Design review of the part built by this model. Coordinates are the model's own, in mm. Face numbers are marked on the shaded views. A direction names the side the tool comes from. Round coordinates to 2 decimals unless told otherwise and drop trailing zeros. Write each loop counter-clockwise with the first axis right and the second up, starting at its lowest first coordinate (ties: lowest second). Pieces come first, ordered by that corner, then holes. Notation, with made-up numbers: (12, 27.25) -> (43, 27.25) arc R4 cw to (43, 32.25) -> close; hole circle Ø11 at (8, 45.5). An arc over 180 degrees is marked (long way). Write item = value, one per line. Start each with the question number.
Item 1: Add section B-B, the plane y = -20. State the section outline as (x, z) points, then the cut area to 3 significant figures.
Item 2: Add section D-D, the plane y = 10. State the section outline as (x, z) points, then the cut area to 3 significant figures.
Item 3: Add section C-C, the plane x = 23. State the section outline as (y, z) points.
Item 4: Add section A-A, the plane x = 0. State the section outline as (y, z) points.
Item 5: For pin 1 Ø6 at (x, z) = (38, 29.5) entering from -Y, flat-tipped, find the tip position at first contact; note if it passes through.
Item 6: To check wall thickness, follow L1, parallel to Z at x = 25, y = -10.5; L2, parallel to Y at x = -21.5, z = 19.5; L3, parallel to Y at x = -13, z = 6.5. State the ranges of each line that lie inside material, in increasing order.
Item 7: Mouldability with a two-part tool opening along Y and no side actions: class the marked faces 1, 2, 3 and 4 as released by +Y, released by -Y, zero draft, split by the parting line, or undercut.
Item 8: Machinability: for the marked faces 5 and 6, which of the approach directions +Z, -Z, +X, -X, +Y, -Y give a long, thin tool a straight path to every point of the face, cutting with its end or side? Answer none if there is none.
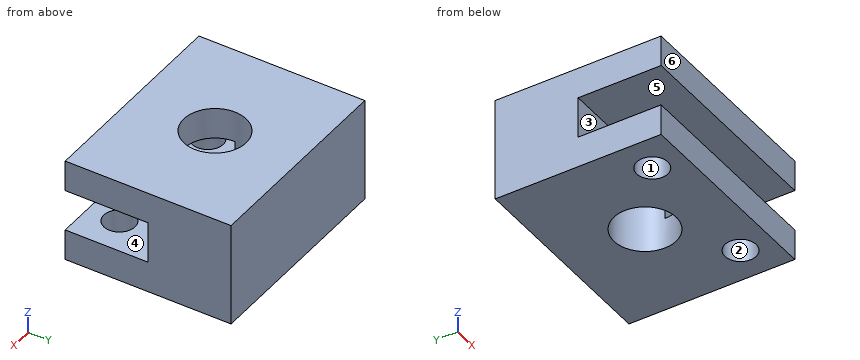
from build123d import *

# Parameters (mm, degrees)
F0_W     = 100
F0_H     = 80
F0_R     = 15
F1_DEPTH = 50
F2_W     = 120
F2_H     = 20
F3_DEPTH = 40
F4_R     = 7.5
F5_DEPTH = 25


with BuildPart() as f1:
    # F0 (on Top) → F1 (new body)
    with BuildSketch(Plane.XY):
        Rectangle(F0_W, F0_H)
        Circle(F0_R, mode=Mode.SUBTRACT)
    extrude(amount=F1_DEPTH)

    # F2 (on face) → F3 (cut)
    with BuildSketch(Plane.XZ.offset(40)):
        with Locations((3.9423131943, 25.000000596)):
            Rectangle(F2_W, F2_H)
    extrude(amount=-F3_DEPTH, mode=Mode.SUBTRACT)

    # F4 (on face) → F5 (cut)
    with BuildSketch(Plane.XY.offset(15.000000596)):
        with Locations((-32.9807698727, -24.8076934367)):
            Circle(F4_R)
        with Locations((32.9807698727, -24.8076934367)):
            Circle(F4_R)
    extrude(amount=-F5_DEPTH, mode=Mode.SUBTRACT)


solid = f1.part
Result set:
q1.outline = (-50, 0) -> (-38.74, 0) -> (-38.74, 15) -> (-50, 15) -> close; (-50, 35) -> (50, 35) -> (50, 50) -> (-50, 50) -> close; (-27.22, 0) -> (27.22, 0) -> (27.22, 15) -> (-27.22, 15) -> close; (38.74, 0) -> (50, 0) -> (50, 15) -> (38.74, 15) -> close
q1.area = 2,650 mm²
q2.outline = (-50, 0) -> (-11.18, 0) -> (-11.18, 50) -> (-50, 50) -> close; (11.18, 0) -> (50, 0) -> (50, 50) -> (11.18, 50) -> close
q2.area = 3,880 mm²
q3.outline = (-40, 0) -> (40, 0) -> (40, 50) -> (-40, 50) -> (-40, 35) -> (0, 35) -> (0, 15) -> (-40, 15) -> close
q4.outline = (-40, 0) -> (-15, 0) -> (-15, 15) -> (-40, 15) -> close; (-40, 35) -> (-15, 35) -> (-15, 50) -> (-40, 50) -> close; (15, 0) -> (40, 0) -> (40, 50) -> (15, 50) -> close
q5.pin_1 = 0
q6.L1 = 0 to 15, 35 to 50
q6.L2 = 0 to 40
q6.L3 = -40 to -7.48, 7.48 to 40
q7.face_1 = undercut
q7.face_2 = undercut
q7.face_3 = released by -Y
q7.face_4 = zero draft
q8.face_5 = +X, -X, -Y
q8.face_6 = +Z, -Z, +X, -X, -Y
